Geometry check sheet. Reference: the model listing, model coordinates, mm. Face numbers are marked on the shaded views. Round coordinates to 2 decimals unless told otherwise and drop trailing zeros. Loops run counter-clockwise (first coordinate to the right, second up) from the corner with the lowest first, then second, coordinate; pieces in that order, holes last. Notation, with made-up numbers: (-10, -13) - (20, -13) arc R20 cw to (20, 1) - close; hole circle Ø10 at (79.25, 78.5). An arc over 180 degrees is marked (long way). Write item = value, one per line.
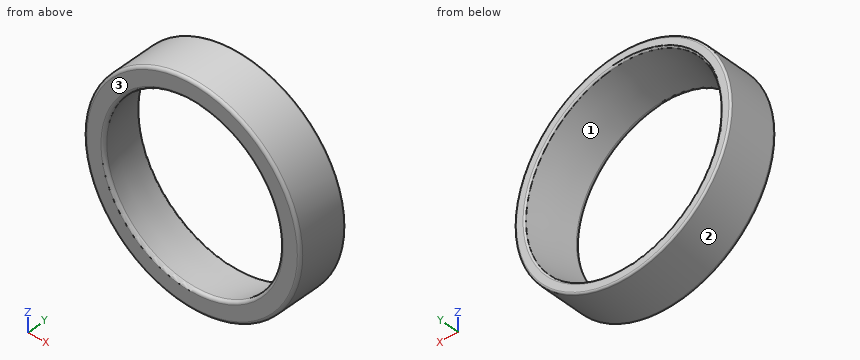
```python
from build123d import *

# Parameters (mm, degrees)
FILLET1_R = 0.5
FILLET3_R = 0.8


with BuildPart() as part:
    # Sketch2 → Revolve1 (revolve)
    with BuildSketch(Plane.XY):
        Polygon((-30.5, 0), (-30.5, 14), (-27.75, 14), (-24.75, 0), align=None)
    revolve(axis=Axis((0, 0, 0), (0, 1, 0)))

    # Fillet1
    fillet1_edges = [part.edges().sort_by_distance(p)[0] for p in [
        (27.75, 14, 0),
        (30.5, 14, 0),
    ]]
    fillet(fillet1_edges, radius=FILLET1_R)

    # Fillet3
    fillet3_edges = [part.edges().sort_by_distance(p)[0] for p in [
        (30.5, 0, 0),
        (24.75, 0, 0),
    ]]
    fillet(fillet3_edges, radius=FILLET3_R)


solid = part.part
```
(1) Section check D-D (y = 11). Enter the section's corners in (x, z).
Answers follow:
outline = circle Ø61 at (0, 0); hole circle Ø54.21 at (0, 0)
(2) Scan lines: L1, parallel to Z at x = -1, y = 12; L2, parallel to Z at x = 1, y = 1.5; L3, parallel to X at y = 5, z = -13. Record each from-to range of solid material in increasing order. Write a range as [from, to].
Answers follow:
L1 = [-30.48, -27.3], [27.3, 30.48]
L2 = [-30.48, -25.05], [25.05, 30.48]
L3 = [-27.59, -22.31], [22.31, 27.59]
(3) Section check A-A (x = 0). Enter the section's corners in (y, z).
Answers follow:
outline = (0, -29.7) arc R0.8 ccw to (0.8, -30.5) - (13.5, -30.5) arc R0.5 ccw to (14, -30) - (14, -28.15) arc R0.5 ccw to (13.6, -27.67) - (0.97, -24.96) arc R0.8 ccw to (0, -25.74) - close; (0, 25.74) arc R0.8 ccw to (0.97, 24.96) - (13.6, 27.67) arc R0.5 ccw to (14, 28.15) - (14, 30) arc R0.5 ccw to (13.5, 30.5) - (0.8, 30.5) arc R0.8 ccw to (0, 29.7) - close
(4) Section check B-B (z = 0). Enter the section's corners in (x, y).
Answers follow:
outline = (-30.5, 0.8) arc R0.8 ccw to (-29.7, 0) - (-25.74, 0) arc R0.8 ccw to (-24.96, 0.97) - (-27.67, 13.6) arc R0.5 ccw to (-28.15, 14) - (-30, 14) arc R0.5 ccw to (-30.5, 13.5) - close; (24.96, 0.97) arc R0.8 ccw to (25.74, 0) - (29.7, 0) arc R0.8 ccw to (30.5, 0.8) - (30.5, 13.5) arc R0.5 ccw to (30, 14) - (28.15, 14) arc R0.5 ccw to (27.67, 13.6) - close
(5) Mould release check, pull along Z, two halves, no side actions. Record for the marked faces 1, 2 and 3: pulls with the +Z half, pulls with the -Z half, needs draft (parallel to the pull), parting line crosses it, or undercut.
Answers follow:
face_1 = undercut
face_2 = parting line crosses it
face_3 = needs draft
(6) Gauge pin test, flat ends, axial feed: pin 1 (2 mm diameter, centred on x = 23, y = 2.5, fed in from -Z); pin 2 (4 mm diameter, centred on x = 4, y = 11.5, fed in from +Z); pin 3 (4 mm diameter, centred on x = -20.5, y = 9.5, fed in from +Z). Record the tip position at first contact, or that the pin passes through.
Answers follow:
pin_1 = -21.12
pin_2 = 30.43
pin_3 = 24.25
(7) Section check C-C (y = 6.5). Enter the section's corners in (x, z), then the cut area to 3 significant figures.
Answers follow:
outline = circle Ø61 at (0, 0); hole circle Ø52.29 at (0, 0)
area = 775 mm²
